CAD build for the part. Positions are in the model's coordinates, mm. A direction names the side the tool comes from. Round coordinates to 2 decimals unless told otherwise and drop trailing zeros. Write each loop counter-clockwise with the first axis right and the second up, starting at its lowest first coordinate (ties: lowest second). Pieces come first, ordered by that corner, then holes. Notation, with made-up numbers: (-25, 36) -> (24, 36) arc R21 ccw to (24, 58) -> close; hole circle Ø2 at (24.25, -31.5). An arc over 180 degrees is marked (long way). Answer in a Markdown table with one row per item. Add a question column.
```python
from build123d import *

# Parameters (mm, degrees)
F1_DEPTH    = 3
F2_DEPTH    = 1
F3_DEPTH    = 3.5
F4_DEPTH    = 1.5
F5_DEPTH    = 1.5
F6_DEPTH    = 25
F7_T1_DEPTH = 38.0035618315
F7_T3_DEPTH = 38.0035618315
F8_SIZE2    = 3.99999
F8_SIZE     = 1.99999
F9_SIZE     = 1.5


# Not quite as in the source:
# - a fillet or chamfer that OpenCascade refuses, or shapes differently, is made with other operations: its cross-section is extruded or revolved along the edge and cut away or added
# - a fillet or chamfer is up to 0.001 mm smaller than in the source, because OpenCascade refuses the exact size


with BuildPart() as f1:
    # F0 (on Top) → F1 (new body)
    with BuildSketch(Plane.XY):
        with BuildLine():
            Line((5.6457948953, 1.625), (7.193747285, 1.625))
            ThreePointArc((7.193747285, 1.625), (-7.375, 0), (7.193747285, -1.625))
            Line((7.193747285, -1.625), (5.6457948953, -1.625))
            ThreePointArc((5.6457948953, -1.625), (-5.875, 0), (5.6457948953, 1.625))
        make_face()
    extrude(amount=F1_DEPTH)

    # F0 (on Top) → F2 (join)
    with BuildSketch(Plane.XY):
        with BuildLine():
            Line((2.3717082451, 1.625), (5.6457948953, 1.625))
            ThreePointArc((5.6457948953, 1.625), (-5.875, 0), (5.6457948953, -1.625))
            Line((5.6457948953, -1.625), (2.3717082451, -1.625))
            ThreePointArc((2.3717082451, -1.625), (-2.875, 0), (2.3717082451, 1.625))
        make_face()
        with BuildLine():
            Line((0, 1.625), (2.3717082451, 1.625))
            ThreePointArc((2.3717082451, 1.625), (-2.875, 0), (2.3717082451, -1.625))
            Line((2.3717082451, -1.625), (0, -1.625))
            ThreePointArc((0, -1.625), (-1.625, 0), (0, 1.625))
        make_face()
    extrude(amount=F2_DEPTH)

    # F0 (on Top) → F3 (join)
    with BuildSketch(Plane.XY):
        with BuildLine():
            Line((5.6457948953, 1.625), (7.193747285, 1.625))
            ThreePointArc((7.193747285, 1.625), (-7.375, 0), (7.193747285, -1.625))
            Line((7.193747285, -1.625), (5.6457948953, -1.625))
            ThreePointArc((5.6457948953, -1.625), (-5.875, 0), (5.6457948953, 1.625))
        make_face()
        with BuildLine():
            Line((2.3717082451, 1.625), (5.6457948953, 1.625))
            ThreePointArc((5.6457948953, 1.625), (-5.875, 0), (5.6457948953, -1.625))
            Line((5.6457948953, -1.625), (2.3717082451, -1.625))
            ThreePointArc((2.3717082451, -1.625), (-2.875, 0), (2.3717082451, 1.625))
        make_face()
    extrude(amount=-F3_DEPTH)

    # F0 (on Top) → F4 (join)
    with BuildSketch(Plane.XY):
        with BuildLine():
            Line((7.193747285, 1.625), (9.3599879808, 1.625))
            ThreePointArc((9.3599879808, 1.625), (6.1160649114, 7.2693706743), (0, 9.5))
            ThreePointArc((0, 9.5), (-9.5, 0), (0, -9.5))
            ThreePointArc((0, -9.5), (6.1160649114, -7.2693706743), (9.3599879808, -1.625))
            Line((9.3599879808, -1.625), (7.193747285, -1.625))
            ThreePointArc((7.193747285, -1.625), (-7.375, 0), (7.193747285, 1.625))
        make_face()
    extrude(amount=-F4_DEPTH)

    # F0 (on Top) → F5 (join)
    with BuildSketch(Plane.XY):
        with BuildLine():
            ThreePointArc((0, -9.5), (-9.5, 0), (0, 9.5))
            Line((0, 9.5), (0, 11.5))
            ThreePointArc((0, 11.5), (-11.5, 0), (0, -11.5))
            Line((0, -11.5), (0, -9.5))
        make_face()
    extrude(amount=-F5_DEPTH)

    # F0 (on Top) → F6 (join)
    with BuildSketch(Plane.XY):
        with BuildLine():
            ThreePointArc((0, -9.5), (-9.5, 0), (0, 9.5))
            Line((0, 9.5), (0, 11.5))
            ThreePointArc((0, 11.5), (-11.5, 0), (0, -11.5))
            Line((0, -11.5), (0, -9.5))
        make_face()
    extrude(amount=F6_DEPTH)

    # F7: chamfer of 7 on 2 edges, made by hand

    # F7_s2 → F7_t1 (cut)
    with BuildSketch(Plane.XZ.offset(-8.5017809158)):
        Polygon((-7, 25), (0, 18), (0, 25), align=None)
    extrude(amount=F7_T1_DEPTH, mode=Mode.SUBTRACT)

    # F7_s4 → F7_t3 (cut)
    with BuildSketch(Plane.XZ.offset(-29.5017809158)):
        Polygon((0, 18), (-7, 25), (0, 25), align=None)
    extrude(amount=F7_T3_DEPTH, mode=Mode.SUBTRACT)

    # F8 (size 2 and 4 in the source; OpenCascade refuses exactly that, so slightly less here)
    f8_edges = [f1.edges().sort_by_distance(p)[0] for p in [
        (-7.375, 0, -3.5),
    ]]
    f8_side = f1.faces().sort_by_distance((-7.375, 0, -2.5))[0]
    chamfer(f8_edges, length=F8_SIZE, length2=F8_SIZE2, reference=f8_side)

    # F9
    f9_edges = [f1.edges().sort_by_distance(p)[0] for p in [
        (-11.5, 0, -1.5),
    ]]
    chamfer(f9_edges, length=F9_SIZE)


solid = f1.part
```
Item 1: Saw through at C-C on z = 10.5. Give the cut face in (x, y).
Item 2: Drill centre lines: probe 1 along Y at (x, z) = (-3.75, 7.25); probe 2 along Z at (x, y) = (-9, 3.75); probe 3 along Y at (x, z) = (-2.5, 7.25). Where is each one in solid material? Low to high.
Item 3: Saw through at A-A on z = 0.5. Give the cut face in (x, y) (3 decimals).
Item 4: Two-plate mould, pull along X, no slides. Class faces 4 (the flat face through (-3, 10, 21)), 5 (the conical face through (-3.57, 0.15, -3.4)), 6 (the cylindrical face through (-7.37, 0.3, 1.52)), 7 (the flat face through (-7, -3, -1.5)): +X half, -X half, draft (parallel to the pull), parting line (faces both ways), or undercut.
Item 5: Pin check, flat tips, straight feed: pin 1 (12 mm diameter, centred on y = -8, z = 9.5, fed in from -X); pin 2 (12 mm diameter, centred on x = -8.5, z = 2.5, fed in from +Y) (3 decimals); pin 3 (1 mm diameter, centred on y = -10, z = 5.5, fed in from +X). Stop position of each tip, or through.
Item 6: Tool access for faces 1 (the flat face through (-2, 0, 0)), 2 (the flat face through (-1.5, -1.2, 1)), 3 (the flat face through (-6, 2, 3)): list every direction of +Z, -Z, +X, -X, +Y, -Y with a clear straight run to the whole face (end or side of a thin tool).
Recorded:
| question | item | result |
|---|---|---|
| 1 | outline | (0, -11.5) -> (0, -9.5) arc R9.5 cw to (0, 9.5) -> (0, 11.5) arc R11.5 ccw to start |
| 2 | probe 1 | -10.87 to -8.73, 8.73 to 10.87 |
| 2 | probe 2 | -1.5 to 25 |
| 2 | probe 3 | -11.22 to -9.17, 9.17 to 11.22 |
| 3 | outline | (0, -11.5) -> (0, -9.5) arc R9.5 cw to (0, 9.5) -> (0, 11.5) arc R11.5 ccw to start; (0, -1.625) arc R1.625 cw to (0, 1.625) -> (7.194, 1.625) arc R7.375 ccw (long way) to (7.194, -1.625) -> close |
| 4 | face 4 | +X half |
| 4 | face 5 | parting line |
| 4 | face 6 | undercut |
| 4 | face 7 | draft |
| 5 | pin 1 | x = -11.32 |
| 5 | pin 2 | y = 11.225 |
| 5 | pin 3 | x = 0 |
| 6 | face 1 | -Z |
| 6 | face 2 | +Z |
| 6 | face 3 | +Z, +X |
